Source: CAD feature listing. Evaluate the final solid. Frame: model axes, mm. A direction names the side the tool comes from. Give positions to 0.01 mm unless a question says otherwise; leave off trailing zeros. Return JSON: item names as keys, results as strings.
from build123d import *

# Parameters (mm, degrees)
SKETCH11_R       = 2
SIZE_4X4_1_DEPTH = 280


with BuildPart() as part:
    # Sketch11 → Size 4X4 (1) (new body)
    with BuildSketch(Plane(origin=(0, 0, 0), x_dir=(0, 0, -1), z_dir=(1, 0, 0))):
        with BuildLine():
            Line((-3, 9.2), (-3, 8.8))
            ThreePointArc((-3, 8.8), (-3.234314575, 8.234314575), (-3.8, 8))
            Line((-3.8, 8), (-6.585786438, 8))
            Line((-6.585786438, 8), (-2.820101013, 4.234314575))
            ThreePointArc((-2.820101013, 4.234314575), (-2.560562334, 4.060896374), (-2.254415588, 4))
            Line((-2.254415588, 4), (2.254415588, 4))
            ThreePointArc((2.254415588, 4), (2.560562334, 4.060896374), (2.820101013, 4.234314575))
            Line((2.820101013, 4.234314575), (6.585786438, 8))
            Line((6.585786438, 8), (3.8, 8))
            ThreePointArc((3.8, 8), (3.234314575, 8.234314575), (3, 8.8))
            Line((3, 8.8), (3, 9.2))
            ThreePointArc((3, 9.2), (3.234314575, 9.765685425), (3.8, 10))
            Line((3.8, 10), (9.2, 10))
            ThreePointArc((9.2, 10), (9.765685425, 9.765685425), (10, 9.2))
            Line((10, 9.2), (10, 3.8))
            ThreePointArc((10, 3.8), (9.765685425, 3.234314575), (9.2, 3))
            Line((9.2, 3), (8.8, 3))
            ThreePointArc((8.8, 3), (8.234314575, 3.234314575), (8, 3.8))
            Line((8, 3.8), (8, 6.585786438))
            Line((8, 6.585786438), (4.234314575, 2.820101013))
            ThreePointArc((4.234314575, 2.820101013), (4.060896374, 2.560562334), (4, 2.254415588))
            Line((4, 2.254415588), (4, -2.254415588))
            ThreePointArc((4, -2.254415588), (4.060896374, -2.560562334), (4.234314575, -2.820101013))
            Line((4.234314575, -2.820101013), (8, -6.585786438))
            Line((8, -6.585786438), (8, -3.8))
            ThreePointArc((8, -3.8), (8.234314575, -3.234314575), (8.8, -3))
            Line((8.8, -3), (9.2, -3))
            ThreePointArc((9.2, -3), (9.765685425, -3.234314575), (10, -3.8))
            Line((10, -3.8), (10, -9.2))
            ThreePointArc((10, -9.2), (9.765685425, -9.765685425), (9.2, -10))
            Line((9.2, -10), (3.8, -10))
            ThreePointArc((3.8, -10), (3.234314575, -9.765685425), (3, -9.2))
            Line((3, -9.2), (3, -8.8))
            ThreePointArc((3, -8.8), (3.234314575, -8.234314575), (3.8, -8))
            Line((3.8, -8), (6.585786438, -8))
            Line((6.585786438, -8), (2.820101013, -4.234314575))
            ThreePointArc((2.820101013, -4.234314575), (2.560562334, -4.060896374), (2.254415588, -4))
            Line((2.254415588, -4), (-2.254415588, -4))
            ThreePointArc((-2.254415588, -4), (-2.560562334, -4.060896374), (-2.820101013, -4.234314575))
            Line((-2.820101013, -4.234314575), (-6.585786438, -8))
            Line((-6.585786438, -8), (-3.8, -8))
            ThreePointArc((-3.8, -8), (-3.234314575, -8.234314575), (-3, -8.8))
            Line((-3, -8.8), (-3, -9.2))
            ThreePointArc((-3, -9.2), (-3.234314575, -9.765685425), (-3.8, -10))
            Line((-3.8, -10), (-9.2, -10))
            ThreePointArc((-9.2, -10), (-9.765685425, -9.765685425), (-10, -9.2))
            Line((-10, -9.2), (-10, -3.8))
            ThreePointArc((-10, -3.8), (-9.765685425, -3.234314575), (-9.2, -3))
            Line((-9.2, -3), (-8.8, -3))
            ThreePointArc((-8.8, -3), (-8.234314575, -3.234314575), (-8, -3.8))
            Line((-8, -3.8), (-8, -6.585786438))
            Line((-8, -6.585786438), (-4.234314575, -2.820101013))
            ThreePointArc((-4.234314575, -2.820101013), (-4.060896374, -2.560562334), (-4, -2.254415588))
            Line((-4, -2.254415588), (-4, 2.254415588))
            ThreePointArc((-4, 2.254415588), (-4.060896374, 2.560562334), (-4.234314575, 2.820101013))
            Line((-4.234314575, 2.820101013), (-8, 6.585786438))
            Line((-8, 6.585786438), (-8, 3.8))
            ThreePointArc((-8, 3.8), (-8.234314575, 3.234314575), (-8.8, 3))
            Line((-8.8, 3), (-9.2, 3))
            ThreePointArc((-9.2, 3), (-9.765685425, 3.234314575), (-10, 3.8))
            Line((-10, 3.8), (-10, 9.2))
            ThreePointArc((-10, 9.2), (-9.765685425, 9.765685425), (-9.2, 10))
            Line((-9.2, 10), (-3.8, 10))
            ThreePointArc((-3.8, 10), (-3.234314575, 9.765685425), (-3, 9.2))
        make_face()
        Circle(SKETCH11_R, mode=Mode.SUBTRACT)
    extrude(amount=SIZE_4X4_1_DEPTH)


solid = part.part
1. Ray query, probe 1 along Y at (x, z) = (87, 0); probe 2 along Y at (x, z) = (15, -5.75); probe 3 along Z at (x, y) = (186, -5.25). Return the intervals inside material, ascending.
Evaluation:
{"probe 1": "y = -4 to -2, 2 to 4", "probe 2": "y = -10 to -8, -7.16 to -4.34, 4.34 to 7.16, 8 to 10", "probe 3": "z = -10 to -8, -6.66 to -3.84, 3.84 to 6.66, 8 to 10"}
2. Set-up query: faces 1 (the face through (138, 0, 4)), 2 (the face through (138, 0, -4)), 3 (the face through (138, -4, 0)). Return all of +Z, -Z, +X, -X, +Y, -Y with unobstructed straight access to the full face (end or side cutting, diameter ignored); none if empty.
Evaluation:
{"face 1": "+Z, +X, -X", "face 2": "-Z, +X, -X", "face 3": "+X, -X, -Y"}
3. First-contact query: pin 1 (3.5 mm diameter, centred on x = 189, z = 0.5, fed in from +Y); pin 2 (1 mm diameter, centred on x = 231.5, z = 3, fed in from +Y); pin 3 (3.5 mm diameter, centred on x = 173, z = 0.5, fed in from -Y). Flat tips, straight axial feed; report the tip coordinate or a pass-through.
Evaluation:
{"pin 1": "stops at y = 4", "pin 2": "stops at y = 9.94", "pin 3": "stops at y = -4"}
4. Draft query along Z for faces 4 (the face through (0, 2.4, -0.1)), 5 (the face through (138, -7, 10)), 6 (the face through (138, 4, 0)). Return one class per face: pulls with the +Z half, pulls with the -Z half, needs draft (parallel to the pull), parting line crosses it, or undercut.
Evaluation:
{"face 4": "needs draft", "face 5": "pulls with the +Z half", "face 6": "undercut"}
